Can you work these out from the drawing? Everything is in mm from the part's minimum corner. A direction names the side the tool comes from. Give positions to 0.01 mm unless a question says otherwise; leave off trailing zeros. Write each loop counter-clockwise with the first axis right and the second up, starting at its lowest first coordinate (ties: lowest second). Pieces come first, ordered by that corner, then holes. Notation, with made-up numbers: (53.5, 69) - (94.5, 69) arc R36 ccw to (94.5, 103) - close; hole circle Ø7 at (-22.5, 58.5). An arc over 180 degrees is marked (long way). Return JSON: item names as keys, results as strings. Group by question number.
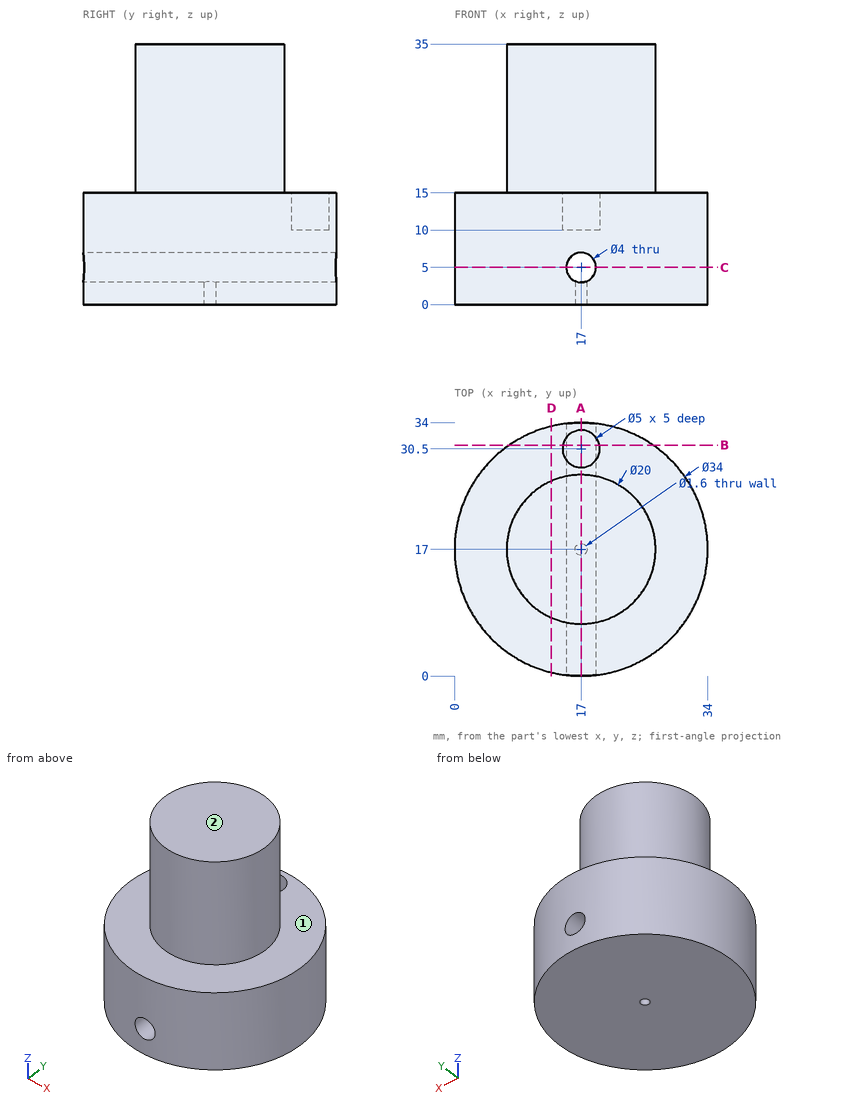
1) Imagine slicing it at C-C, the plane z = 5. Write out the boundary of the cut face in (x, y).
2) Will these pins go through, and if not, where does the flat tip stop? pin 1 Ø4 at (y, z) = (20, 29.5) entering from +X; pin 2 Ø3 at (x, z) = (25.5, 29) entering from +Y; pin 3 Ø2.5 at (x, z) = (17, 5) entering from +Y; pin 4 Ø12 at (y, z) = (17.5, 29.5) entering from +X.
3) Imagine slicing it at B-B, the plane y = 31. Write out the boundary of the cut face in (x, z), and give its area (3 significant figures).
4) On a 3-axis mill with a long thin cutter (end or side, diameter ignored), from which of +Z, -Z, +X, -X, +Y, -Y can I reach the whole of each face in a straight line? I mean the marked faces 1 and 2. Say none if no direction works.
5) Imagine slicing it at D-D, the plane x = 13. Write out the boundary of the cut face in (y, z).
6) Imagine slicing it at A-A, the plane x = 17. Write out the boundary of the cut face in (y, z).
7) I need wall thicknesses on line 1 along Y through (x, z) = (17, 12); line 2 along Z through (x, y) = (17, 21); line 3 along Y through (x, z) = (17, 32). Which ranges of each line are inside material? Lowest first, please.
Resolved:
{
 "1": {"outline": "(15, 0.12) - (15, 33.88) arc R17 ccw to start; (19, 0.12) arc R17 ccw to (19, 33.88) - close"},
 "2": {"pin 1": "x = 26.95", "pin 2": "y = 24.14", "pin 3": "through", "pin 4": "x = 27"},
 "3": {"outline": "(7.36, 0) - (26.64, 0) - (26.64, 15) - (19.45, 15) - (19.45, 10) - (14.55, 10) - (14.55, 15) - (7.36, 15) - close; hole circle Ø4 at (17, 5)", "area": "252 mm^2"},
 "4": {"face 1": "+Z", "face 2": "+Z, +X, -X, +Y, -Y"},
 "5": {"outline": "(0.48, 0) - (33.52, 0) - (33.52, 15) - (26.17, 15) - (26.17, 35) - (7.83, 35) - (7.83, 15) - (0.48, 15) - close"},
 "6": {"outline": "(0, 0) - (16.2, 0) - (16.2, 3) - (0, 3) - close; (0, 7) - (34, 7) - (34, 15) - (33, 15) - (33, 10) - (28, 10) - (28, 15) - (27, 15) - (27, 35) - (7, 35) - (7, 15) - (0, 15) - close; (17.8, 0) - (34, 0) - (34, 3) - (17.8, 3) - close"},
 "7": {"line 1": "0 to 28, 33 to 34", "line 2": "0 to 3, 7 to 35", "line 3": "7 to 27"}
}
